Here's how the part is built. I have some questions about the finished solid (model axes, mm). Coordinates: 2 decimals unless noted, no trailing zeros. Write each loop counter-clockwise with the first axis right and the second up, starting at its lowest first coordinate (ties: lowest second). Pieces come first, ordered by that corner, then holes.
Autodesk Inventor part; units mm, degrees
ref_plane "YZ Plane" through (0, 0, 0) normal (1, 0, 0) x (0, 1, 0)
ref_plane "XZ Plane" through (0, 0, 0) normal (0, 1, 0) x (-1, 0, 0)
ref_plane "XY Plane" through (0, 0, 0) normal (0, 0, 1) x (1, 0, 0)
sketch "Sketch1" plane through (0, 0, 0) normal (0, 0, 1) x (1, 0, 0)
  line L0 (0, 0) -> (170, 0)
  line L1 (170, 0) -> (170, 170)
  line L2 (170, 170) -> (0, 170)
  line L3 (0, 170) -> (0, 0)
  dimension "d0" = 170
  dimension "d1" = 170
extrude "Extrusion1" add sketch "Sketch1" along normal blind 10
sketch "Sketch2" plane through (0, 0, 10) normal (0, 0, 1) x (1, 0, 0)
  line L0 (170, 170) -> (0, 170)
  line L1 (0, 170) -> (0, 155)
  line L2 (0, 170) -> (0, 0)
  line L3 (0, 0) -> (170, 0)
  line L4 (0, 0) -> (0, 15)
  line L5 (0, 15) -> (155, 15)
  line L6 (155, 15) -> (155, 155)
  line L7 (155, 155) -> (15, 155)
  line L8 (15, 155) -> (15, 15)
  line L9 (15, 155) -> (30, 155)
  circle A0 centre (15, 155) radius 7.5
  circle A1 centre (155, 155) radius 7.5
  circle A2 centre (155, 15) radius 7.5
  circle A3 centre (15, 15) radius 7.5
  dimension "d4" = 15
  dimension "d5" = 15
  dimension "d6" = 155
  dimension "d7" = 140
  dimension "d8" = 140
  dimension "d9" = 140
  dimension "d10" = 15
  dimension "d11" = 15
  dimension "d12" = 15
  dimension "d13" = 15
extrude "Extrusion2" cut sketch "Sketch2" against normal blind 10 contours L8 A3 L5 | L5 A3 | L5 A3 L8 | A2 L6 L5 | L5 L6 A2 | A0 L7 L8 | L8 L7 A0 | A1 L7 L6 | L6 L7 A1
sketch "Sketch3" plane through (0, 0, 10) normal (0, 0, 1) x (1, 0, 0)
  line L0 (170, 170) -> (0, 170)
  line L1 (0, 170) -> (85, 170)
  line L2 (85, 170) -> (85, 85)
  circle A0 centre (85, 85) radius 7.5
  point P0 (0, 0)
  dimension "d16" = 85
  dimension "d17" = 85
  dimension "d18" = 15
extrude "Extrusion3" cut sketch "Sketch3" against normal blind 10
sketch "Sketch4" plane through (0, 0, 10) normal (0, 0, 1) x (1, 0, 0)
  line L0 (0, 0) -> (170, 0)
  line L1 (0, 0) -> (85, 0)
  line L2 (85, 0) -> (85, 40)
  circle A0 centre (85, 40) radius 7.5
  dimension "d21" = 85
  dimension "d22" = 40
  dimension "d23" = 15
extrude "Extrusion4" cut sketch "Sketch4" against normal blind 10
properties part number "AZ"
1) I need wall thicknesses on probe 1 along X at (y, z) = (15, 4); probe 2 along Y at (x, z) = (14.5, 5.25); probe 3 along Y at (x, z) = (85, 5.5). Which ranges of each line are inside material? Lowest first, please.
Values follow:
probe 1: x = 0 to 7.5, 22.5 to 147.5, 162.5 to 170
probe 2: y = 0 to 7.52, 22.48 to 147.52, 162.48 to 170
probe 3: y = 0 to 32.5, 47.5 to 77.5, 92.5 to 170
2) We'd pull the mould along X, two halves only. Please class faces 1 (the face through (79.048, 35.436, 5.07)), 2 (the face through (162.154, 157.253, 5.07)), 3 (the face through (86, 170, 5)), 4 (the face through (170, 84, 5)): pulls with the +X half, pulls with the -X half, needs draft (parallel to the pull), parting line crosses it, or undercut.
Values follow:
face 1: undercut
face 2: undercut
face 3: needs draft
face 4: pulls with the +X half
3) Imagine slicing it at B-B on x = 15. Please give me the cut outline in (y, z).
Values follow:
outline: (0, 0) - (7.5, 0) - (7.5, 10) - (0, 10) - close; (22.5, 0) - (147.5, 0) - (147.5, 10) - (22.5, 10) - close; (162.5, 0) - (170, 0) - (170, 10) - (162.5, 10) - close
4) Imagine slicing it at A-A on y = 40. Please give me the cut outline in (x, z), then the cut area to 3 significant figures.
Values follow:
outline: (0, 0) - (77.5, 0) - (77.5, 10) - (0, 10) - close; (92.5, 0) - (170, 0) - (170, 10) - (92.5, 10) - close
area: 1,550 mm2
5) Imagine slicing it at C-C on z = 2.5. Please give me the cut outline in (x, y).
Values follow:
outline: (0, 0) - (170, 0) - (170, 170) - (0, 170) - close; hole circle Ø15 at (15, 15); hole circle Ø15 at (15, 155); hole circle Ø15 at (85, 40); hole circle Ø15 at (85, 85); hole circle Ø15 at (155, 15); hole circle Ø15 at (155, 155)
